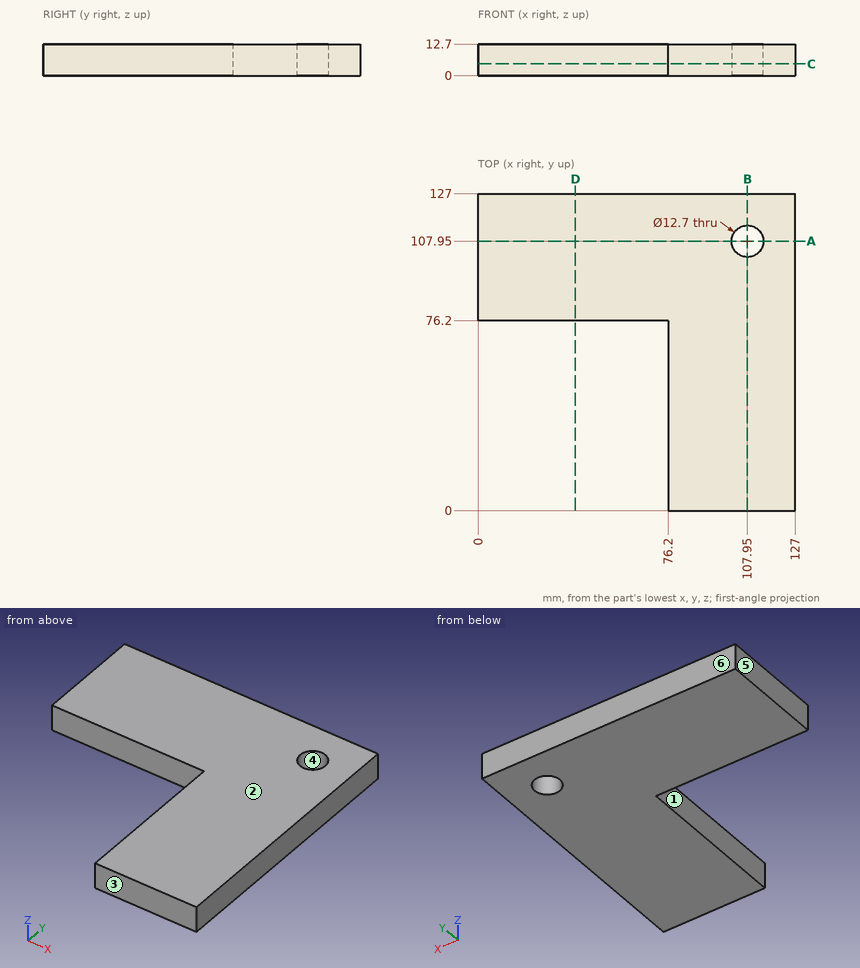
For this review, use the dimensioned drawing (mm, ordinates from the lowest corner) and the shaded views. A direction names the side the tool comes from. Round coordinates to 2 decimals unless told otherwise and drop trailing zeros. Write each loop counter-clockwise with the first axis right and the second up, starting at its lowest first coordinate (ties: lowest second). Pieces come first, ordered by that corner, then holes. Notation, with made-up numbers: (-5.75, -7) -> (41.25, -7) arc R24 ccw to (41.25, 23) -> close; hole circle Ø4 at (9, 88). An arc over 180 degrees is marked (long way). Use CSV: the item, a comma, the result in double quotes.
(1) To check wall thickness, follow L1, parallel to Y at x = 107.95, z = 8.75; L2, parallel to X at y = 52, z = 10. State the ranges of each line that lie inside material, in increasing order. Write a range as [from, to].
Computed values:
L1,"[0, 101.6], [114.3, 127]"
L2,"[76.2, 127]"
(2) Clearance check with flat-ended pins moving along their axes: P1, Ø1.5, axis at y = 109.5, z = 8.5, coming from the -X side; P2, Ø1, axis at y = 13.5, z = 11.5, coming from the -X side. State where each tip first meets the part, or that it passes through.
Computed values:
P1,"x = 0"
P2,"x = 76.2"
(3) For the marked faces 1 and 2, list the 3-axis set-ups (+Z, -Z, +X, -X, +Y, -Y) from which the entire face can be reached by the end or side of a thin tool; tool diameter is ignored.
Computed values:
face 1,"+Z, -Z, -X, -Y"
face 2,"+Z, +X, -X, +Y, -Y"
(4) Consider section A-A, the plane y = 107.95. Give the boundary of the cut face in (x, z).
Computed values:
outline,"(0, 0) -> (101.6, 0) -> (101.6, 12.7) -> (0, 12.7) -> close; (114.3, 0) -> (127, 0) -> (127, 12.7) -> (114.3, 12.7) -> close"
(5) Consider section D-D, the plane x = 39. Give the boundary of the cut face in (y, z), plus the area to 3 significant figures.
Computed values:
outline,"(76.2, 0) -> (127, 0) -> (127, 12.7) -> (76.2, 12.7) -> close"
area,"645 mm²"
(6) Consider section C-C, the plane z = 4.75. Give the boundary of the cut face in (x, y), plus the area to 3 significant figures.
Computed values:
outline,"(0, 76.2) -> (76.2, 76.2) -> (76.2, 0) -> (127, 0) -> (127, 127) -> (0, 127) -> close; hole circle Ø12.7 at (107.95, 107.95)"
area,"10,200 mm²"
(7) Draft analysis for pull direction Y (two halves, no side actions). For the marked faces 3, 4, 5 and 6, state which applies: +Y half, -Y half, draft (parallel to the pull), parting line (faces both ways), or undercut.
Computed values:
face 3,"-Y half"
face 4,"undercut"
face 5,"draft"
face 6,"+Y half"
